The figure shows three views and two pictorial views of one solid part (mm, origin at its lowest corner). Answer the questions. Coordinates: 2 decimals unless noted, no trailing zeros. Order: outer loops, then holes, each group sorted by start corner. A loop starts at its lowest first (then second) coordinate and runs counter-clockwise, first axis right, second up. Notation, with made-up numbers: M 6.25,46.5 L 37.25,46.5 A26 ccw 37.25,72.5 Z; hole C 87,-17 d3. An arc over 180 degrees is marked long. Write item = value, one per line. Start each with the question number.
Q1. Straight lines are drawn through the part: line 1 along Z through (x, y) = (6.5, 258) (1 decimal); line 2 along Y through (x, z) = (10, 47.5); line 3 along Z through (x, y) = (24.5, 82) (1 decimal). For each, find the intervals that lie inside material, in ascending order.
Q2. Find section A-A on y = 264. Give the vertices of the cut face in (x, z) (1 decimal), and give its area (4 significant figures).
Q3. Find section B-B on x = 20.5. Give the vertices of the cut face in (y, z) (1 decimal).
Q4. Determine the mould class of the marked faces 1, 2 and 3 for opening direction X: released by +X, released by -X, zero draft, split by the parting line, or undercut.
Q5. Find section C-C on z = 34.5. Give the vertices of the cut face in (x, y), and give its area (3 significant figures).
Q6. Each of these flat-tipped pins is pushed along its axis until it touches: P1, Ø4, axis at x = 7.5, z = 33.5, coming from the +Y side; P2, Ø2, axis at x = 21, y = 98, coming from the -Z side; P3, Ø6, axis at x = 15.5, z = 33, coming from the +Y side. Where does it stop, or does it pass through?
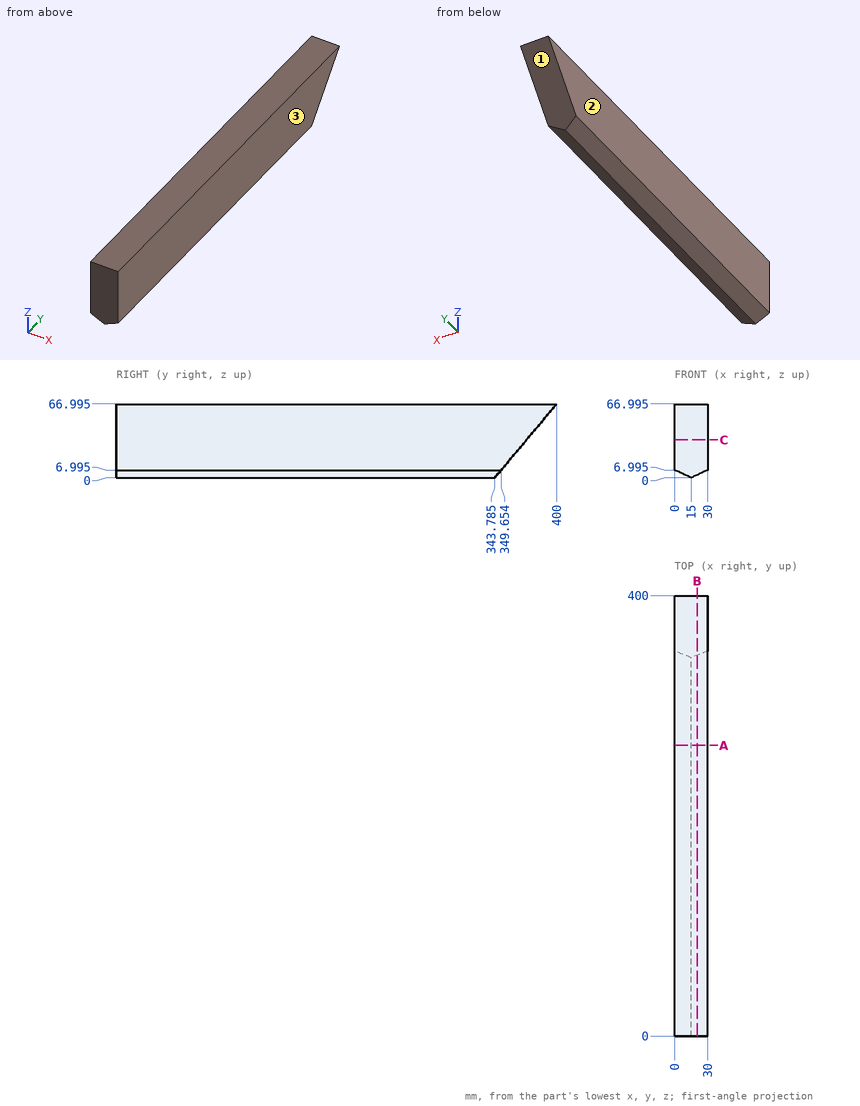
Findings below:
q1.line_1 = 4 to 67
q1.line_2 = 0 to 383.64
q1.line_3 = 4.4 to 67
q2.outline = M 0,7 L 15,0 L 30,7 L 30,67 L 0,67 Z
q2.area = 1,905 mm^2
q3.outline = M 0,2.6 L 345.9,2.6 L 400,67 L 0,67 Z
q4.face_1 = zero draft
q4.face_2 = released by -X
q4.face_3 = released by +X
q5.outline = M 0,0 L 30,0 L 30,372.73 L 0,372.73 Z
q5.area = 11,200 mm^2
q6.P1 = 373.57
q6.P2 = 2.33
q6.P3 = 373.99
